from build123d import *

# Parameters (mm, degrees)
MODEL_R             = 1.5
MODEL_R_2           = 1.6
BOSS_EXTRUDE1_DEPTH = 6.25


with BuildPart() as part:
    # Model → Boss-Extrude1 (new body)
    with BuildSketch(Plane.XY):
        Polygon((4.400116, 111), (45.400116, 70), (61.514718626, 70), (102.514718626, 111), (107.485169777, 111), (111, 107.485169777), (111, 102.514718626), (73, 64.514718626), (73, 41.666961), (111, 3.666961), (111, -3.666961), (73, -41.666961), (73, -64.514718626), (111, -102.514718626), (111, -107.485169777), (107.485169777, -111), (102.514718626, -111), (61.514718626, -70), (45.400116, -70), (4.400116, -111), (-4.400116, -111), (-45.400116, -70), (-66.514718626, -70), (-107.514718626, -111), (-112.485169777, -111), (-116, -107.485169777), (-116, -102.514718626), (-89, -75.514718626), (-89, -62), (-98.5, -52.5), (-98.5, -21.239105), (-116, -3.739105), (-116, 3.739105), (-98.5, 21.239105), (-98.5, 52.5), (-89, 62), (-89, 75.514718626), (-116, 102.514718626), (-116, 107.485169777), (-112.485169777, 111), (-107.514718626, 111), (-66.514718626, 70), (-45.400116, 70), (-4.400116, 111), align=None)
        with Locations((0, -105)):
            Circle(MODEL_R, mode=Mode.SUBTRACT)
        with Locations((0, 105)):
            Circle(MODEL_R, mode=Mode.SUBTRACT)
        with Locations((105, -105)):
            Circle(MODEL_R, mode=Mode.SUBTRACT)
        with Locations((-110, 105)):
            Circle(MODEL_R, mode=Mode.SUBTRACT)
        with Locations((105, 105)):
            Circle(MODEL_R, mode=Mode.SUBTRACT)
        with Locations((-110, 0)):
            Circle(MODEL_R, mode=Mode.SUBTRACT)
        Circle(MODEL_R, mode=Mode.SUBTRACT)
        with Locations((105, 0)):
            Circle(MODEL_R, mode=Mode.SUBTRACT)
        with Locations((76.5, 0)):
            Circle(MODEL_R_2, mode=Mode.SUBTRACT)
        with Locations((96.5, 0)):
            Circle(MODEL_R_2, mode=Mode.SUBTRACT)
        with Locations((-73.5, 35)):
            Circle(MODEL_R_2, mode=Mode.SUBTRACT)
        with Locations((-73.5, -35)):
            Circle(MODEL_R_2, mode=Mode.SUBTRACT)
        with Locations((-93.5, 35)):
            Circle(MODEL_R_2, mode=Mode.SUBTRACT)
        with Locations((-93.5, -35)):
            Circle(MODEL_R_2, mode=Mode.SUBTRACT)
        with Locations((-110, -105)):
            Circle(MODEL_R, mode=Mode.SUBTRACT)
        with Locations((1.5, -19.5)):
            Circle(MODEL_R, mode=Mode.SUBTRACT)
        with Locations((1.5, 19.5)):
            Circle(MODEL_R, mode=Mode.SUBTRACT)
        Polygon((-18, -7.97703218), (-38.02296782, -28), (-55.000029993, -28), (-78.5, -4.5), (-78.5, 4.5), (-55.000029993, 28), (-38.02296782, 28), (-18, 7.97703218), align=None, mode=Mode.SUBTRACT)
        Polygon((71.5, 25.014709), (60.98529, 35.529449), (44.014709, 35.529449), (17, 8.51474), (17, -8.51474), (44.014709, -35.529449), (60.98529, -35.529449), (71.5, -25.014709), align=None, mode=Mode.SUBTRACT)
        Polygon((-37, 61.415771), (-37, 44.566314), (-20.433686, 28), (19.51474, 28), (36, 44.48526), (36, 62.429580116), (3.682617, 94.746963116), (-3.682617, 94.733154), align=None, mode=Mode.SUBTRACT)
        Polygon((-37, -61.415771), (-37, -44.566314), (-20.433686, -28), (19.51474, -28), (36, -44.48526), (36, -62.429580116), (3.682617, -94.746963116), (-3.682617, -94.733154), align=None, mode=Mode.SUBTRACT)
        with BuildLine():
            Line((-78.499999987, 41.75), (-78.499999987, 28.25))
            Line((-78.499999987, 28.25), (-77.999999987, 27.75))
            Line((-77.999999987, 27.75), (-77.899999843, 27.75))
            ThreePointArc((-77.899999843, 27.75), (-74.899999843, 24.75), (-77.899999843, 21.75))
            Line((-77.899999843, 21.75), (-89.100000157, 21.75))
            ThreePointArc((-89.100000157, 21.75), (-92.100000157, 24.75), (-89.100000157, 27.75))
            Line((-89.100000157, 27.75), (-89.000000013, 27.75))
            Line((-89.000000013, 27.75), (-88.500000013, 28.25))
            Line((-88.500000013, 28.25), (-88.500000013, 41.75))
            Line((-88.500000013, 41.75), (-89.000000013, 42.25))
            Line((-89.000000013, 42.25), (-89.100000157, 42.25))
            ThreePointArc((-89.100000157, 42.25), (-92.100000157, 45.25), (-89.100000157, 48.25))
            Line((-89.100000157, 48.25), (-77.899999843, 48.25))
            ThreePointArc((-77.899999843, 48.25), (-74.899999843, 45.25), (-77.899999843, 42.25))
            Line((-77.899999843, 42.25), (-77.999999987, 42.25))
            Line((-77.999999987, 42.25), (-78.499999987, 41.75))
        make_face(mode=Mode.SUBTRACT)
        with BuildLine():
            Line((91.500000013, 6.75), (91.500000013, -6.75))
            Line((91.500000013, -6.75), (92.000000013, -7.25))
            Line((92.000000013, -7.25), (92.100000157, -7.25))
            ThreePointArc((92.100000157, -7.25), (95.100000157, -10.25), (92.100000157, -13.25))
            Line((92.100000157, -13.25), (80.899999843, -13.25))
            ThreePointArc((80.899999843, -13.25), (77.899999843, -10.25), (80.899999843, -7.25))
            Line((80.899999843, -7.25), (80.999999987, -7.25))
            Line((80.999999987, -7.25), (81.499999987, -6.75))
            Line((81.499999987, -6.75), (81.499999987, 6.75))
            Line((81.499999987, 6.75), (80.999999987, 7.25))
            Line((80.999999987, 7.25), (80.899999843, 7.25))
            ThreePointArc((80.899999843, 7.25), (77.899999843, 10.25), (80.899999843, 13.25))
            Line((80.899999843, 13.25), (92.100000157, 13.25))
            ThreePointArc((92.100000157, 13.25), (95.100000157, 10.25), (92.100000157, 7.25))
            Line((92.100000157, 7.25), (92.000000013, 7.25))
            Line((92.000000013, 7.25), (91.500000013, 6.75))
        make_face(mode=Mode.SUBTRACT)
        with BuildLine():
            Line((-78.499999987, -28.25), (-78.499999987, -41.75))
            Line((-78.499999987, -41.75), (-77.999999987, -42.25))
            Line((-77.999999987, -42.25), (-77.899999843, -42.25))
            ThreePointArc((-77.899999843, -42.25), (-74.899999843, -45.25), (-77.899999843, -48.25))
            Line((-77.899999843, -48.25), (-89.100000157, -48.25))
            ThreePointArc((-89.100000157, -48.25), (-92.100000157, -45.25), (-89.100000157, -42.25))
            Line((-89.100000157, -42.25), (-89.000000013, -42.25))
            Line((-89.000000013, -42.25), (-88.500000013, -41.75))
            Line((-88.500000013, -41.75), (-88.500000013, -28.25))
            Line((-88.500000013, -28.25), (-89.000000013, -27.75))
            Line((-89.000000013, -27.75), (-89.100000157, -27.75))
            ThreePointArc((-89.100000157, -27.75), (-92.100000157, -24.75), (-89.100000157, -21.75))
            Line((-89.100000157, -21.75), (-77.899999843, -21.75))
            ThreePointArc((-77.899999843, -21.75), (-74.899999843, -24.75), (-77.899999843, -27.75))
            Line((-77.899999843, -27.75), (-77.999999987, -27.75))
            Line((-77.999999987, -27.75), (-78.499999987, -28.25))
        make_face(mode=Mode.SUBTRACT)
    extrude(amount=BOSS_EXTRUDE1_DEPTH)


solid = part.part
Input: part model. Units: mm. Frame: model coordinates. A direction names the side the tool comes from. Give positions to 0.01 mm unless a question says otherwise; leave off trailing zeros. Write each loop counter-clockwise with the first axis right and the second up, starting at its lowest first coordinate (ties: lowest second). Pieces come first, ordered by that corner, then holes. Notation, with made-up numbers: M 43,-39 L 96,-39 A6 ccw 96,-34 Z; hole C 13,86 d11. An arc over 180 degrees is marked long. Use one line per item in the form item = value.
1. Reachability of faces 1 (the face through (-102.689, -89.204, 3.081)), 2 (the face through (91.734, -83.249, 3.081)), 3 (the face through (-88.5, -35, 3)), 4 (the face through (-56, -70, 3)) from +Z, -Z, +X, -X, +Y, -Y: full face, straight path, thin tool, end or side. Return the list, or none.
Outcome:
face_1 = +Z, -Z, -X
face_2 = +Z, -Z, +X
face_3 = +Z, -Z
face_4 = +Z, -Z, -Y
2. Mould query, pull axis Y, two halves, no side actions, for faces 5 (the face through (-86.728, -90.213, 3.081)), 6 (the face through (-25.2, 90.2, 3.1)), 7 (the face through (-92.1, -24.8, 3.1)), 8 (the face through (-116, 105, 3)). Classes: released by +Y, released by -Y, zero draft, split by the parting line, or undercut.
Outcome:
face_5 = released by -Y
face_6 = released by +Y
face_7 = undercut
face_8 = zero draft
3. Cut plane A-A on y = -85.5. Return loops of the section in (x, z).
Outcome:
outline = M -98.99,0 L -82.01,0 L -82.01,6.25 L -98.99,6.25 Z; M -29.9,0 L -12.92,0 L -12.92,6.25 L -29.9,6.25 Z; M 12.93,0 L 29.9,0 L 29.9,6.25 L 12.93,6.25 Z; M 77.01,0 L 93.99,0 L 93.99,6.25 L 77.01,6.25 Z
4. Cut plane C-C on z = 3.5. State how many separate pieces and enclosed holes the cut face has, and give its area (3 significant figures).
Outcome:
separate_pieces = 1
enclosed_holes = 24
area = 19,000 mm²
5. Ray query, L1, parallel to X at y = 47, z = 2.5; L2, parallel to X at y = 10, z = 5; L3, parallel to X at y = 78, z = 5.25. Return the intervals inside material, ascending.
Outcome:
L1 = -98.5 to -91.54, -75.46 to -37, 36 to 73
L2 = -109.74 to -73, -20.02 to 18.49, 71.5 to 77.91, 95.09 to 104.67
L3 = -91.49 to -74.51, -37.4 to -20.42, 20.43 to 37.4, 69.51 to 86.49
6. Cut plane B-B on x = -59. Return loops of the section in (y, z).
Outcome:
outline = M -70,0 L -24,0 L -24,6.25 L -70,6.25 Z; M 24,0 L 70,0 L 70,6.25 L 24,6.25 Z
7. First-contact query: P1, Ø3, axis at x = -73.5, y = -35, coming from the +Z side; P2, Ø3, axis at x = -58.5, z = 3.5, coming from the +Y side; P3, Ø3, axis at x = -83, z = 2, coming from the +Y side; P4, Ø3, axis at x = -39.5, z = 1, coming from the -Y side. Flat tips, straight axial feed; report the tip coordinate or a pass-through.
Outcome:
P1 = through
P2 = 70
P3 = 87.99
P4 = -77.4
